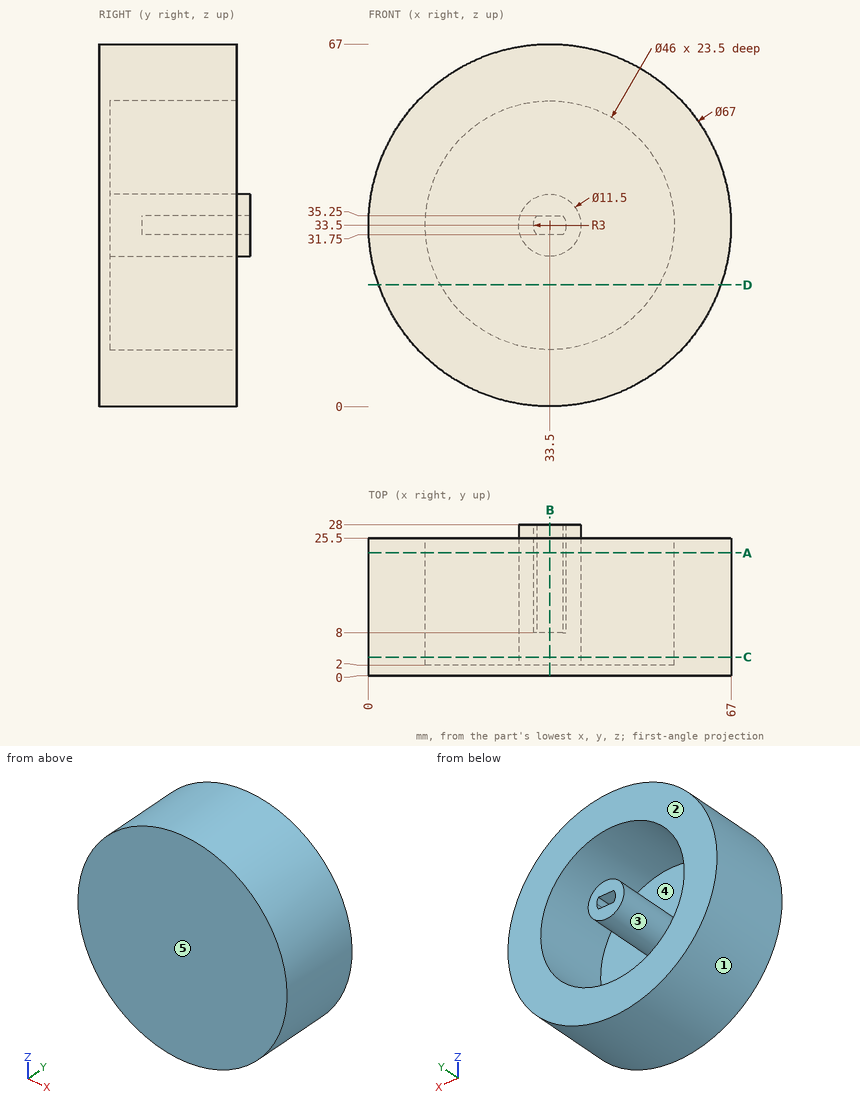
Verification items for this drawing (mm, ordinates from the low corner). A direction names the side the tool comes from. Give positions to 0.01 mm unless a question says otherwise; leave off trailing zeros. Loops run counter-clockwise (first coordinate to the right, second up) from the corner with the lowest first, then second, coordinate; pieces in that order, holes last. Notation, with made-up numbers: M -14,48.5 L 36,48.5 A29 ccw 36,83.5 Z; hole C 36,-35.5 d11. An arc over 180 degrees is marked long. Write item = value, one per line. Start each with the question number.
1. Go/stop test with flat-tipped pins: P1, Ø20, axis at x = 49, z = 48, coming from the +Y side; P2, Ø2, axis at x = 41, y = 16.5, coming from the +Z side; P3, Ø2.5, axis at x = 32.5, y = 16, coming from the +Z side; P4, Ø1, axis at y = 18, z = 28.5, coming from the +X side. Record where each tip stops, or that it passes through.
2. Section check A-A, the plane y = 22.75. Enter the section's corners in (x, z).
3. Section check D-D, the plane z = 22.5. Enter the section's corners in (x, y), plus the area to 3 significant figures.
4. Tool access check on the marked faces 4 and 5. Record the directions out of +Z, -Z, +X, -X, +Y, -Y that give a thin tool (end or side, any length) a straight path to the whole face; none if there is none.
5. Draft check along X on the marked faces 1, 2 and 3. Enter one of: +X half, -X half, draft (parallel to the pull), parting line (faces both ways), or undercut.
6. Section check C-C, the plane y = 3.5. Enter the section's corners in (x, z), plus the area to 3 significant figures.
7. Thickness scan on probe 1 along X at (y, z) = (17.75, 33.5); probe 2 along X at (y, z) = (3.5, 29.5); probe 3 along X at (y, z) = (13.75, 31). Record the ranges inside material, lowest first.
8. Section check B-B, the plane x = 33.5. Enter the section's corners in (y, z), plus the area to 4 significant figures.
Values follow:
q1.P1 = 25.5
q1.P2 = 66.36
q1.P3 = 67
q1.P4 = 66.7
q2.outline = C 33.5,33.5 d67; C 33.5,33.5 d11.5; hole C 33.5,33.5 d46; hole M 31.06,31.75 L 35.94,31.75 A3 ccw 35.94,35.25 L 31.06,35.25 A3 ccw Z
q3.outline = M 1.86,0 L 65.14,0 L 65.14,25.5 L 53.7,25.5 L 53.7,2 L 13.3,2 L 13.3,25.5 L 1.86,25.5 Z
q3.area = 664 mm^2
q4.face_4 = +Y
q4.face_5 = +Z, -Z, +X, -X, -Y
q5.face_1 = parting line
q5.face_2 = draft
q5.face_3 = undercut
q6.outline = C 33.5,33.5 d67; C 33.5,33.5 d11.5; hole C 33.5,33.5 d46
q6.area = 1,970 mm^2
q7.probe_1 = 0 to 10.5, 27.75 to 30.5, 36.5 to 39.25, 56.5 to 67
q7.probe_2 = 0.24 to 10.85, 29.37 to 37.63, 56.15 to 66.76
q7.probe_3 = 0.09 to 10.64, 28.32 to 38.68, 56.36 to 66.91
q8.outline = M 0,0 L 25.5,0 L 25.5,10.5 L 2,10.5 L 2,27.75 L 28,27.75 L 28,31.75 L 8,31.75 L 8,35.25 L 28,35.25 L 28,39.25 L 2,39.25 L 2,56.5 L 25.5,56.5 L 25.5,67 L 0,67 Z
q8.area = 856.5 mm^2
